Design review of the part built by this model. Coordinates are the model's own, in mm. A direction names the side the tool comes from. Coordinates: 2 decimals unless noted, no trailing zeros. Loops run counter-clockwise (first coordinate to the right, second up) from the corner with the lowest first, then second, coordinate; pieces in that order, holes last. Notation, with made-up numbers: M 57.25,-20 L 74.25,-20 A26 ccw 74.25,-6 Z; hole C 54,26.25 d6. An arc over 180 degrees is marked long. Put each result on its own line as item: value. Start each with the question number.
(1) The part is to be moulded in two halves that separate along Y. For faces 1 (the cylindrical face through (-10.1, 7.7, 22)), 2 (the cylindrical face through (14.605, -22.908, -28.531)), 3 (the flat face through (18, -11, -112.126)), say which applies: +Y half, -Y half, draft (parallel to the pull), parting line (faces both ways), or undercut.
(2) Clearance check with flat-ended pins moving along their axes: pin 1 (8 mm diameter, centred on y = 3.5, z = 61.5, fed in from +X); pin 2 (5 mm diameter, centred on x = 26, z = 174, fed in from +Y); pin 3 (10 mm diameter, centred on x = -2.5, y = -30.5, fed in from -Z). State where each tip first meets the part, or that it passes through.
(3) Take a section at B-B, the plane z = 77. Give the boundary of the cut face in (x, y), then the cut area to 3 significant figures.
(4) For probe 1 along Y at (x, z) = (0, 147); probe 2 along Y at (x, z) = (0, 33); probe 3 along Z at (x, y) = (23, 28.5), list the stretches that pass through material, from the lowest coordinate up. Write a range as [from, to].
(5) For faces 4 (the flat face through (10, 10, 264.038)), 5 (the flat face through (26, 18, 61.488)), list the 3-axis set-ups (+Z, -Z, +X, -X, +Y, -Y) from which the entire face can be reached by the end or side of a thin tool; tool diameter is ignored.
(6) Take a section at A-A, the plane z = -108. Give the boundary of the cut face in (x, y).
```python
from build123d import *


with BuildPart() as part:
    # Sketch1 → Revolve1 (revolve)
    with BuildSketch(Plane(origin=(0, 0, 0), x_dir=(0, 0, -1), z_dir=(1, 0, 0)), mode=Mode.PRIVATE) as revolve1_sk:
        Polygon((-264.03808, 12.7), (213.40064, 12.7), (213.40064, 16.31696), (166.38016, 16.31696), (166.38016, 19.93392), (112.12576, 19.93392), (112.12576, 23.55088), (57.87136, 23.55088), (57.87136, 27.16784), (0, 27.16784), (0, 30.7848), (-61.48832, 30.7848), (-61.48832, 34.40176), (-122.97664, 34.40176), (-122.97664, 38.01872), (-188.08192, 38.01872), (-188.08192, 41.63568), (-224.25152, 41.63568), (-224.25152, 48.8696), (-264.03808, 48.8696), (-264.03808, 38.01872), align=None)
    revolve(revolve1_sk.sketch.rotate(Axis((0, 0, 19.904928919), (0, 0, -1)), 90), axis=Axis((0, 0, 19.904928919), (0, 0, -1)))


solid = part.part
```
Computed values:
1. face 1: undercut
1. face 2: parting line
1. face 3: draft
2. pin 1: stops at x = 34.4
2. pin 2: stops at y = 29.89
2. pin 3: stops at z = -57.87
3. outline: C 0,0 d68.8; hole C 0,0 d25.4
3. area: 3,210 mm^2
4. probe 1: y = [-38.02, -12.7], [12.7, 38.02]
4. probe 2: y = [-30.78, -12.7], [12.7, 30.78]
4. probe 3: z = [122.98, 264.04]
5. face 4: +Z, +X, -X, +Y, -Y
5. face 5: -Z
6. outline: C 0,0 d47.1; hole C 0,0 d25.4
